Check sheet for the drawn part. Datum: minimum x, y, z corner. Units: mm. Give positions to 0.01 mm unless a question says otherwise; leave off trailing zeros. Loops run counter-clockwise (first coordinate to the right, second up) from the corner with the lowest first, then second, coordinate; pieces in that order, holes last. Notation, with made-up numbers: (28, 84) - (69, 84) arc R30 cw to (69, 110) - close; hole circle Ø6 at (55, -1.5). An arc over 180 degrees is marked (long way). Use a Markdown table: item, result. Add a question column.
1. Cross-section at D-D on x = 16. Enter the section's corners in (y, z).
2. Cross-section at A-A on y = 79. Enter the section's corners in (x, z).
3. Cross-section at B-B on z = 1. Enter the section's corners in (x, y), and give its area (3 significant figures).
4. Depth check by flat-ended pin: P1, Ø3.5, axis at x = 28, z = 1, coming from the -Y side; P2, Ø4, axis at x = 53.5, y = 40.75, coming from the -Z side; P3, Ø0.9, axis at y = 73.5, z = 1.5, coming from the +X side; P4, Ø1.8, axis at x = 2.5, y = 2.5, coming from the +Z side. Enter the tip coordinate at first touch or a pass-through.
5. Cross-section at C-C on x = 2.5. Enter the section's corners in (y, z), and give its area (3 significant figures).
6. Draft check along X on the marked faces 1 and 2. Enter one of: pulls with the +X half, pulls with the -X half, needs draft (parallel to the pull), parting line crosses it, or undercut.
7. Material ranges on L1, parallel to X at y = 79, z = 5.05; L2, parallel to Y at x = 2.5, z = 4.4; L3, parallel to Y at x = 42, z = 0.8, recorded low to high.
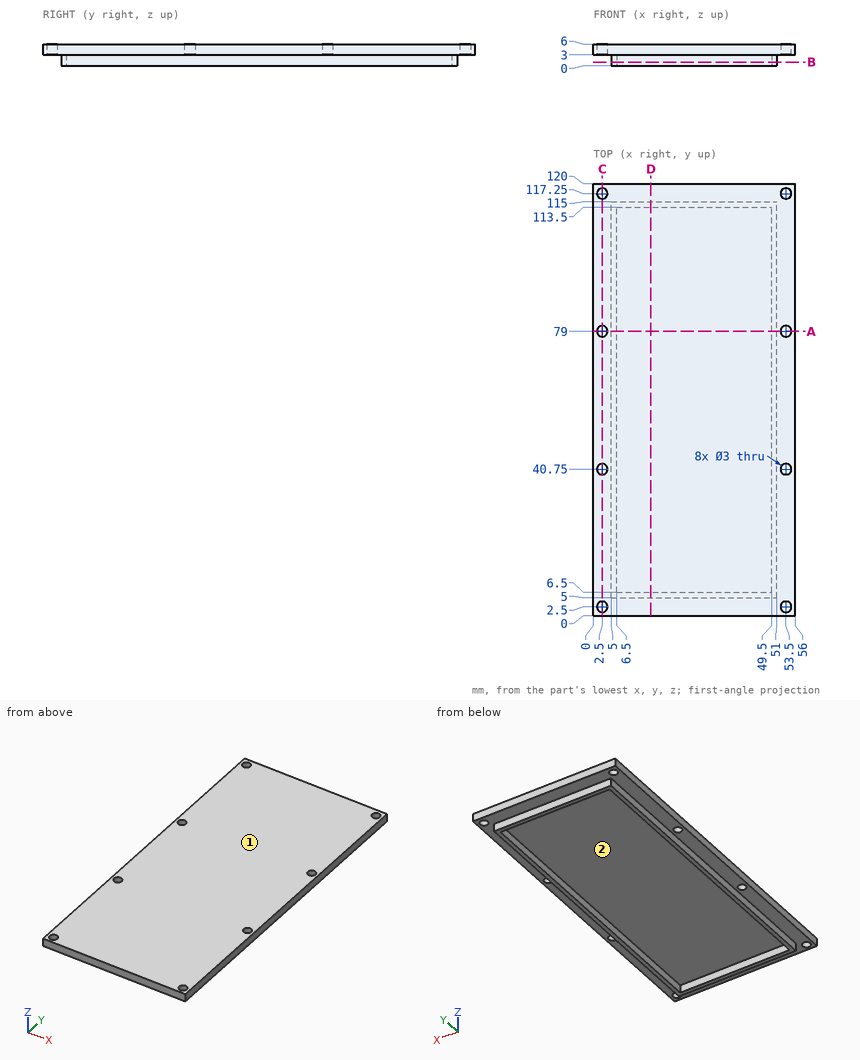
Values found:
| question | item | result |
|---|---|---|
| 1 | outline | (0, 3) - (5, 3) - (5, 0) - (6.5, 0) - (6.5, 3) - (113.5, 3) - (113.5, 0) - (115, 0) - (115, 3) - (120, 3) - (120, 6) - (0, 6) - close |
| 2 | outline | (0, 3) - (1, 3) - (1, 6) - (0, 6) - close; (4, 3) - (5, 3) - (5, 0) - (6.5, 0) - (6.5, 3) - (49.5, 3) - (49.5, 0) - (51, 0) - (51, 3) - (52, 3) - (52, 6) - (4, 6) - close; (55, 3) - (56, 3) - (56, 6) - (55, 6) - close |
| 3 | outline | (5, 5) - (51, 5) - (51, 115) - (5, 115) - close; hole (6.5, 6.5) - (49.5, 6.5) - (49.5, 113.5) - (6.5, 113.5) - close |
| 3 | area | 459 mm2 |
| 4 | P1 | stops at y = 5 |
| 4 | P2 | stops at z = 3 |
| 4 | P3 | stops at x = 51 |
| 4 | P4 | passes through |
| 5 | outline | (0, 3) - (1, 3) - (1, 6) - (0, 6) - close; (4, 3) - (39.25, 3) - (39.25, 6) - (4, 6) - close; (42.25, 3) - (77.5, 3) - (77.5, 6) - (42.25, 6) - close; (80.5, 3) - (115.75, 3) - (115.75, 6) - (80.5, 6) - close; (118.75, 3) - (120, 3) - (120, 6) - (118.75, 6) - close |
| 5 | area | 324 mm2 |
| 6 | face 1 | needs draft |
| 6 | face 2 | undercut |
| 7 | L1 | x = 0 to 1, 4 to 52, 55 to 56 |
| 7 | L2 | y = 0 to 1, 4 to 39.25, 42.25 to 77.5, 80.5 to 115.75, 118.75 to 120 |
| 7 | L3 | y = 5 to 6.5, 113.5 to 115 |
